```python
from build123d import *

# Parameters (mm, degrees)
F1_DEPTH    = 10
F2_T1_DEPTH = 15.2616750858


# Not quite as in the source:
# - a fillet or chamfer that OpenCascade refuses, or shapes differently, is made with other operations: its cross-section is extruded or revolved along the edge and cut away or added


with BuildPart() as f1:
    # F0 (on Top) → F1 (new body)
    with BuildSketch(Plane.XY):
        Polygon((4.7359447583, 0), (-2.6640552417, 0), (-2.4023754605, 4.9931476738), (-3.4023754605, 4.9931476738), (-3.716463021, -1), (5.683536979, -1), (5.474264977, 4.9931476738), (4.474264977, 4.9931476738), align=None)
    extrude(amount=F1_DEPTH)

    # F2: fillet of radius 1 on 2 edges, made by hand

    # F2_s2 → F2_t1 (cut)
    with BuildSketch(Plane.XY.offset(-2.6308375429)):
        with BuildLine():
            ThreePointArc((5.474264977, 4.9931476738), (4.78436631, 4.6632120235), (4.5293399365, 3.9422548452))
            Line((4.5293399365, 3.9422548452), (4.474264977, 4.9931476738))
            Line((4.474264977, 4.9931476738), (5.474264977, 4.9931476738))
        make_face()
        with BuildLine():
            ThreePointArc((-2.4574504199, 3.9422548452), (-2.7124767935, 4.6632120235), (-3.4023754605, 4.9931476738))
            Line((-3.4023754605, 4.9931476738), (-2.4023754605, 4.9931476738))
            Line((-2.4023754605, 4.9931476738), (-2.4574504199, 3.9422548452))
        make_face()
    extrude(amount=F2_T1_DEPTH, mode=Mode.SUBTRACT)


solid = f1.part
```
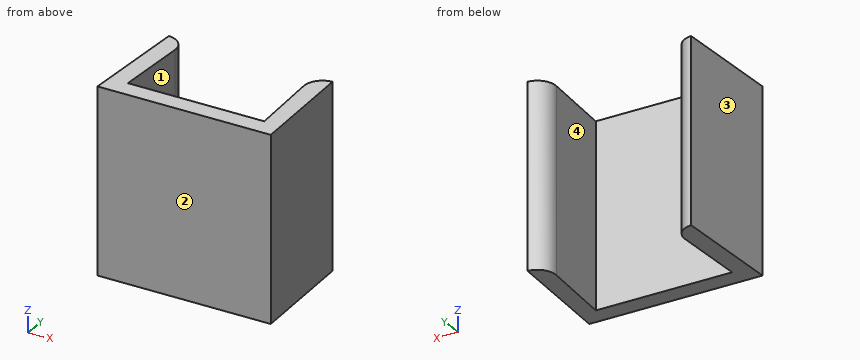
The model under review builds one solid part; all positions refer to its coordinate system, in mm. Face numbers are marked on the shaded views. Give positions to 0.01 mm unless a question says otherwise; leave off trailing zeros. Write each loop counter-clockwise with the first axis right and the second up, starting at its lowest first coordinate (ties: lowest second). Pieces come first, ordered by that corner, then holes.
(1) To check wall thickness, follow L1, parallel to Y at x = 2.5, z = 5.25; L2, parallel to X at y = 2.45, z = 4.5; L3, parallel to X at y = 0.85, z = 3. State the ranges of each line that lie inside material, in increasing order.
(2) Consider section C-C, the plane x = 0.5. Give the boundary of the cut face in (y, z).
(3) Consider section D-D, the plane y = 4.45. Give the boundary of the cut face in (x, z), and give its area (3 significant figures).
(4) Consider section A-A, the plane y = 1.6. Give the boundary of the cut face in (x, z), and give its area (3 significant figures).
(5) Consider section B-B, the plane z = 8.5. Give the boundary of the cut face in (x, y).
(6) The part is to be moulded in two halves that separate along Y. For the marked faces 1, 2, 3 and 4, say which applies: released by +Y, released by -Y, zero draft, split by the parting line, or undercut.
(7) For P1, Ø1.5, axis at y = 2.5, z = 4.5, coming from the +X side; P2, Ø2, axis at x = -1.5, y = 4, coming from the +Z side, all flat-tipped, find the tip position at first contact; note any pin that passes through.
Returned:
1. L1: y = -1 to 0
1. L2: x = -3.54 to -2.54, 4.61 to 5.56
1. L3: x = -3.62 to -2.62, 4.69 to 5.62
2. outline: (-1, 0) - (0, 0) - (0, 10) - (-1, 10) - close
3. outline: (-3.43, 0) - (-2.57, 0) - (-2.57, 10) - (-3.43, 10) - close; (4.64, 0) - (5.49, 0) - (5.49, 10) - (4.64, 10) - close
3. area: 17.2 mm2
4. outline: (-3.58, 0) - (-2.58, 0) - (-2.58, 10) - (-3.58, 10) - close; (4.65, 0) - (5.59, 0) - (5.59, 10) - (4.65, 10) - close
4. area: 19.4 mm2
5. outline: (-3.72, -1) - (5.68, -1) - (5.47, 4.99) arc R1 ccw to (4.53, 3.94) - (4.74, 0) - (-2.66, 0) - (-2.46, 3.94) arc R1 ccw to (-3.4, 4.99) - close
6. face 1: undercut
6. face 2: released by -Y
6. face 3: released by +Y
6. face 4: undercut
7. P1: stops at x = 5.59
7. P2: stops at z = 10
